The model under review builds one solid part; all positions refer to its coordinate system, in mm. Face numbers are marked on the shaded views. A direction names the side the tool comes from. Round coordinates to 2 decimals unless told otherwise and drop trailing zeros. Write each loop counter-clockwise with the first axis right and the second up, starting at its lowest first coordinate (ties: lowest second). Pieces come first, ordered by that corner, then holes.
Item 1: To check wall thickness, follow L1, parallel to Z at x = 53, y = 12; L2, parallel to X at y = 13.5, z = -40; L3, parallel to X at y = 5.5, z = 3. State the ranges of each line that lie inside material, in increasing order.
Item 2: Clearance check with flat-ended pins moving along their axes: pin 1 Ø2 at (x, y) = (33.5, 8) entering from +Z; pin 2 Ø4 at (y, z) = (13.5, -40.5) entering from -X; pin 3 Ø1.6 at (x, y) = (-6, 11) entering from -Z. State where each tip first meets the part, or that it passes through.
Item 3: Add section C-C (y = 9.75). Give the boundary of the cut face in (x, z), plus the area to 3 significant figures.
Item 4: Add section D-D (z = -22.5). Give the boundary of the cut face in (x, y).
Item 5: Add section B-B (z = -4). Give the boundary of the cut face in (x, y), plus the area to 4 significant figures.
Item 6: Add section A-A (x = 1). Give the boundary of the cut face in (y, z).
Item 7: Machinability: for the marked faces 5, 6, 7, 8 and 9, which of the approach directions +Z, -Z, +X, -X, +Y, -Y give a long, thin tool a straight path to every point of the face, cutting with its end or side? Answer none if there is none.
Item 8: Draft analysis for pull direction Z (two halves, no side actions). For the marked faces 1, 2, 3 and 4, state which applies: +Z half, -Z half, draft (parallel to the pull), parting line (faces both ways), or undercut.
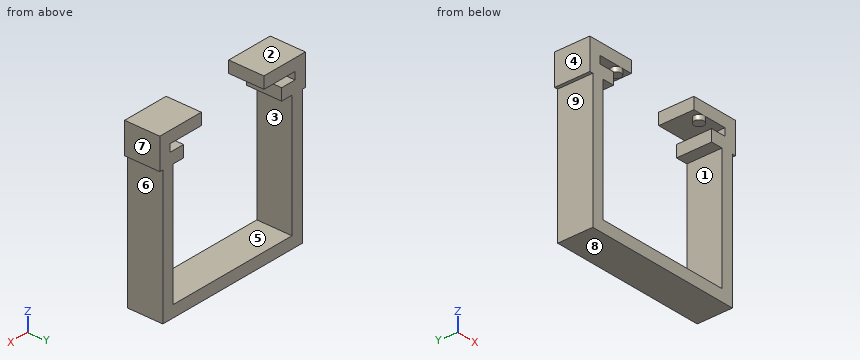
```python
from build123d import *

# Parameters (mm, degrees)
EXTRUDE_1_DEPTH = 15
SKETCH_3_W      = 5
SKETCH_3_H      = 5
EXTRUDE_3_DEPTH = 15
SKETCH_4_R      = 2.15
EXTRUDE_4_DEPTH = 2


with BuildPart() as part:
    # Эскиз1 → Вытянуть1 (new body)
    with BuildSketch(Plane(origin=(0, 0, 0), x_dir=(1, 0, 0), z_dir=(0, 1, 0))):
        Polygon((-5, 5), (-5, 62.3), (62.3, 62.3), (62.3, 5), (63.75, 5), (63.75, -8.2), (43.75, -8.2), (43.75, -3.2), (58.75, -3.2), (58.75, 0), (57.3, 0), (57.3, 57.3), (0, 57.3), (0, 0), (-1.45, 0), (-1.45, -3.2), (13.55, -3.2), (13.55, -8.2), (-6.45, -8.2), (-6.45, 5), align=None)
    extrude(amount=EXTRUDE_1_DEPTH)

    # Эскиз3 → Вытянуть3 (add)
    with BuildSketch(Plane(origin=(0, 0, 0), x_dir=(1, 0, 0), z_dir=(0, 1, 0))):
        with Locations((2.5, 2.5)):
            Rectangle(SKETCH_3_W, SKETCH_3_H)
        with Locations((54.8, 2.5)):
            Rectangle(SKETCH_3_W, SKETCH_3_H)
    extrude(amount=EXTRUDE_3_DEPTH)

    # Эскиз4 → Вытянуть4 (add)
    with BuildSketch(Plane(origin=(0, 0, 3.2), x_dir=(-1, 0, 0), z_dir=(0, 0, -1))):
        with Locations(Location((-8.65, 2.15, 0), (0, 0, 270))):
            Circle(SKETCH_4_R)
        with Locations(Location((-48.65, 2.15, 0), (0, 0, 270))):
            Circle(SKETCH_4_R)
    extrude(amount=EXTRUDE_4_DEPTH)


solid = part.part
```
Numbers:
1. L1: z = -62.3 to -57.3, -5 to 0, 3.2 to 8.2
1. L2: x = -5 to 0, 57.3 to 62.3
1. L3: x = -6.45 to -1.45, 58.75 to 63.75
2. pin 1: stops at z = -57.3
2. pin 2: stops at x = -5
2. pin 3: stops at z = -5
3. outline: (-6.45, -5) - (-5, -5) - (-5, -62.3) - (62.3, -62.3) - (62.3, -5) - (63.75, -5) - (63.75, 8.2) - (43.75, 8.2) - (43.75, 3.2) - (58.75, 3.2) - (58.75, 0) - (52.3, 0) - (52.3, -5) - (57.3, -5) - (57.3, -57.3) - (0, -57.3) - (0, -5) - (5, -5) - (5, 0) - (-1.45, 0) - (-1.45, 3.2) - (13.55, 3.2) - (13.55, 8.2) - (-6.45, 8.2) - close
3. area: 1,210 mm2
4. outline: (-5, 0) - (0, 0) - (0, 15) - (-5, 15) - close; (57.3, 0) - (62.3, 0) - (62.3, 15) - (57.3, 15) - close
5. outline: (-6.45, 0) - (5, 0) - (5, 15) - (-6.45, 15) - close; (52.3, 0) - (63.75, 0) - (63.75, 15) - (52.3, 15) - close
5. area: 343.5 mm2
6. outline: (0, -62.3) - (15, -62.3) - (15, -57.3) - (0, -57.3) - close; (0, -5) - (15, -5) - (15, 0) - (0, 0) - close; (0, 3.2) - (15, 3.2) - (15, 8.2) - (0, 8.2) - close
7. face 5: +Y, -Y
7. face 6: -Z, +X, +Y, -Y
7. face 7: +Z, -Z, +X, +Y, -Y
7. face 8: -Z, +X, -X, +Y, -Y
7. face 9: -Z, -X, +Y, -Y
8. face 1: undercut
8. face 2: +Z half
8. face 3: undercut
8. face 4: draft
